```python
from build123d import *
from OCP.BRepFilletAPI import BRepFilletAPI_MakeChamfer

# Parameters (mm, degrees)
SKETCH1_W                 = 30
SKETCH1_H                 = 30
SKETCH1_R                 = 9.525
BOSS_EXTRUDE1_DEPTH       = 15
CHAMFER2_SIZE             = 0.5
CHAMFER2_SIZE2            = 0.866025404
CHAMFER3_SIZE             = 0.5
M3X0_5_TAPPED_HOLE1_D     = 2.5
M3X0_5_TAPPED_HOLE1_DEPTH = 6
M3X0_5_TAPPED_HOLE1_TIP   = 0.751075774


with BuildPart() as part:
    # Sketch1 → Boss-Extrude1 (new, symmetric)
    with BuildSketch(Plane.XY):
        Rectangle(SKETCH1_W, SKETCH1_H)
        Circle(SKETCH1_R, mode=Mode.SUBTRACT)
    extrude(amount=BOSS_EXTRUDE1_DEPTH, both=True)

    # Chamfer2: one chamfer whose edges measure the first distance from different faces: ONE call of the kernel's chamfer builder (chamfer() names one face for all edges)
    chamfer2_edges_1 = [part.edges().sort_by_distance(p)[0] for p in [
        (-9.525, 0, -15),
    ]]
    chamfer2_side_1 = [part.faces().sort_by_distance(p)[0] for p in [
        (0, -14.575735931, -15),
    ]]
    chamfer2_edges_2 = [part.edges().sort_by_distance(p)[0] for p in [
        (-9.525, 0, 15),
    ]]
    chamfer2_side_2 = [part.faces().sort_by_distance(p)[0] for p in [
        (-9.525, 0, 0),
    ]]
    chamfer2 = BRepFilletAPI_MakeChamfer(part.part.solid().wrapped)
    for e in chamfer2_edges_1:
        chamfer2.Add(CHAMFER2_SIZE, CHAMFER2_SIZE2, e.wrapped, chamfer2_side_1[0].wrapped)  # the first distance lies on this face
    for e in chamfer2_edges_2:
        chamfer2.Add(CHAMFER2_SIZE, CHAMFER2_SIZE2, e.wrapped, chamfer2_side_2[0].wrapped)  # the first distance lies on this face
    add(Compound.cast(chamfer2.Shape()), mode=Mode.REPLACE)

    # Chamfer3
    chamfer3_edges = [part.edges().sort_by_distance(p)[0] for p in [
        (0, 15, -15),
        (0, -15, -15),
    ]]
    chamfer(chamfer3_edges, length=CHAMFER3_SIZE)

    # M3x0.5 Tapped Hole1
    with Locations(Plane(origin=(0, 15, 0), x_dir=(1, 0, 0), z_dir=(0, 1, 0))):
        with Locations((-10, 0), (10, 0), (0, 0), (-10, 10), (-10, -10), (10, 10), (10, -10), (0, 10), (0, -10)):
            Hole(M3X0_5_TAPPED_HOLE1_D / 2, depth=M3X0_5_TAPPED_HOLE1_DEPTH)
            with Locations((0, 0, -(M3X0_5_TAPPED_HOLE1_DEPTH + M3X0_5_TAPPED_HOLE1_TIP / 2))):  # 118° drill point
                Cone(0, M3X0_5_TAPPED_HOLE1_D / 2, M3X0_5_TAPPED_HOLE1_TIP, mode=Mode.SUBTRACT)


solid = part.part
```
Model file for the job. Use its own axes, mm. A direction names the side the tool comes from. Coordinates: 2 decimals unless noted, no trailing zeros. Write each loop counter-clockwise with the first axis right and the second up, starting at its lowest first coordinate (ties: lowest second). Pieces come first, ordered by that corner, then holes. Notation, with made-up numbers: (55.25, -4) - (78.25, -4) arc R20 ccw to (78.25, 17) - close; hole circle Ø6 at (67, 50). An arc over 180 degrees is marked (long way). One line per item, written item: value. Start each with the question number.
1. Tool access for faces 1 (the cylindrical face through (0.16, 12.18, -11.24)), 2 (the flat face through (-4, 10, 15)): list every direction of +Z, -Z, +X, -X, +Y, -Y with a clear straight run to the whole face (end or side of a thin tool).
2. Flat gauge pins, fed straight in: pin 1 (1.5 mm diameter, centred on x = 0, z = 10, fed in from +Y); pin 2 (11.5 mm diameter, centred on x = 0, y = 0, fed in from +Z); pin 3 (2 mm diameter, centred on x = -10, z = 0, fed in from +Y). Where does each tip first touch, or does it go through?
3. Slice it at B-B (z = -4.5). Write the cut outline in (x, y) (3 decimals), plus the area to 3 significant figures.
4. Slice it at A-A (y = 0). Write the cut outline in (x, z) (3 decimals), plus the area to 3 significant figures.
5. Probe line 1 (Z direction, x = -10, y = 11); line 2 (Y direction, x = 0.25, z = -13.25). List the from-to ranges inside material, lowest first. Write a range as from..to.
Answers below:
1. face 1: +Y
1. face 2: +Z, +X, -X, +Y, -Y
2. pin 1: stops at y = -9.5
2. pin 2: passes through
2. pin 3: stops at y = 8.85
3. outline: (-15, -15) - (15, -15) - (15, 15) - (-15, 15) - close; hole circle Ø19.05 at (0, 0)
3. area: 615 mm^2
4. outline: (-15, -15) - (-10.025, -15) - (-9.525, -14.134) - (-9.525, 14.5) - (-10.391, 15) - (-15, 15) - close; (9.525, -14.134) - (10.025, -15) - (15, -15) - (15, 15) - (10.391, 15) - (9.525, 14.5) - close
4. area: 328 mm^2
5. line 1: z = -15..-11.25, -8.75..-1.25, 1.25..8.75, 11.25..15
5. line 2: y = -15..-9.52, 9.52..15
